The listing builds one solid part. Answer for the finished solid, in the listing's coordinates (mm). Face numbers are marked on the shaded views. Give positions to 0.01 mm unless a question says otherwise; leave off trailing zeros. Write each loop counter-clockwise with the first axis right and the second up, starting at its lowest first coordinate (ties: lowest second). Pieces come first, ordered by that corner, then holes. Notation, with made-up numbers: (-13.75, 81.25) - (28.25, 81.25) arc R7 cw to (28.25, 87.25) - close; hole circle Ø2 at (0.25, -1). An arc over 180 degrees is marked (long way). One line per item, written item: value. Start each with the question number.
from build123d import *

# Parameters (mm, degrees)
F0_W     = 177.8
F0_H     = 127
F1_DEPTH = 127
F2_T     = -12.7
F3_DEPTH = 25.4
F4_R     = 25.4


with BuildPart() as f1:
    # F0 (on Top) → F1 (new body)
    with BuildSketch(Plane.XY):
        with Locations((88.9, -63.5)):
            Rectangle(F0_W, F0_H)
    extrude(amount=F1_DEPTH)

    # F2
    f2_openings = [f1.faces().sort_by_distance(p)[0] for p in [
        (88.9, -63.5, 127),
    ]]
    offset(amount=F2_T, openings=f2_openings)

    # F3 (add): a face of the model
    f3_faces = [f1.faces().sort_by_distance(p)[0] for p in [
        (88.9, -63.5, 12.7),
    ]]
    extrude(f3_faces, amount=F3_DEPTH)

    # F4
    f4_edges = [f1.edges().sort_by_distance(p)[0] for p in [
        (177.8, 0, 63.5),
        (177.8, -127, 63.5),
        (0, 0, 63.5),
        (0, -127, 63.5),
    ]]
    fillet(f4_edges, radius=F4_R)


solid = f1.part
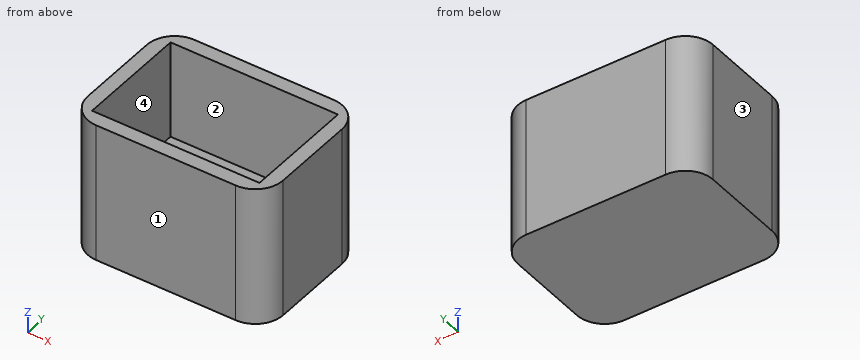
Item 1: Find section A-A on y = -74. Determine the outline of the cut face in (x, z), plus the area to 3 significant figures.
Item 2: Straight lines are drawn through the part: line 1 along Y through (x, z) = (67, 68); line 2 along X through (y, z) = (-39, 112); line 3 along Z through (x, y) = (26.5, -58.5). For each, find the intervals that lie inside material, in ascending order.
Item 3: The mould has two halves that part along Y. Classify the marked faces 1, 2, 3 and 4: +Y half, -Y half, draft (parallel to the pull), parting line (faces both ways), or undercut.
Item 4: Find section B-B on z = 71. Determine the outline of the cut face in (x, y), plus the area to 3 significant figures.
Item 5: Each of these flat-tipped pins is pushed along its axis until it touches: pin 1 Ø10 at (x, y) = (46.5, -39.5) entering from +Z; pin 2 Ø5 at (x, y) = (57.5, -44.5) entering from -Z; pin 3 Ø1.5 at (y, z) = (-23.5, 108) entering from +X. Where does it stop, or does it pass through?
Item 6: Find section C-C on x = 67. Determine the outline of the cut face in (y, z), plus the area to 3 significant figures.
Values:
1. outline: (0, 0) - (177.8, 0) - (177.8, 127) - (165.1, 127) - (165.1, 38.1) - (12.7, 38.1) - (12.7, 127) - (0, 127) - close
1. area: 9,030 mm^2
2. line 1: -127 to -114.3, -12.7 to 0
2. line 2: 0 to 12.7, 165.1 to 177.8
2. line 3: 0 to 38.1
3. face 1: -Y half
3. face 2: undercut
3. face 3: draft
3. face 4: undercut
4. outline: (0, -101.6) arc R25.4 ccw to (25.4, -127) - (152.4, -127) arc R25.4 ccw to (177.8, -101.6) - (177.8, -25.4) arc R25.4 ccw to (152.4, 0) - (25.4, 0) arc R25.4 ccw to (0, -25.4) - close; hole (12.7, -114.3) - (165.1, -114.3) - (165.1, -12.7) - (12.7, -12.7) - close
4. area: 6,540 mm^2
5. pin 1: z = 38.1
5. pin 2: z = 0
5. pin 3: x = 177.77
6. outline: (-127, 0) - (0, 0) - (0, 127) - (-12.7, 127) - (-12.7, 38.1) - (-114.3, 38.1) - (-114.3, 127) - (-127, 127) - close
6. area: 7,100 mm^2
